Drawing for the job (mm, zero at the part's lowest x, y, z). A direction names the side the tool comes from. Give positions to 0.01 mm unless a question says otherwise; leave off trailing zeros. Write each loop counter-clockwise with the first axis right and the second up, starting at its lowest first coordinate (ties: lowest second). Pieces come first, ordered by that corner, then holes.
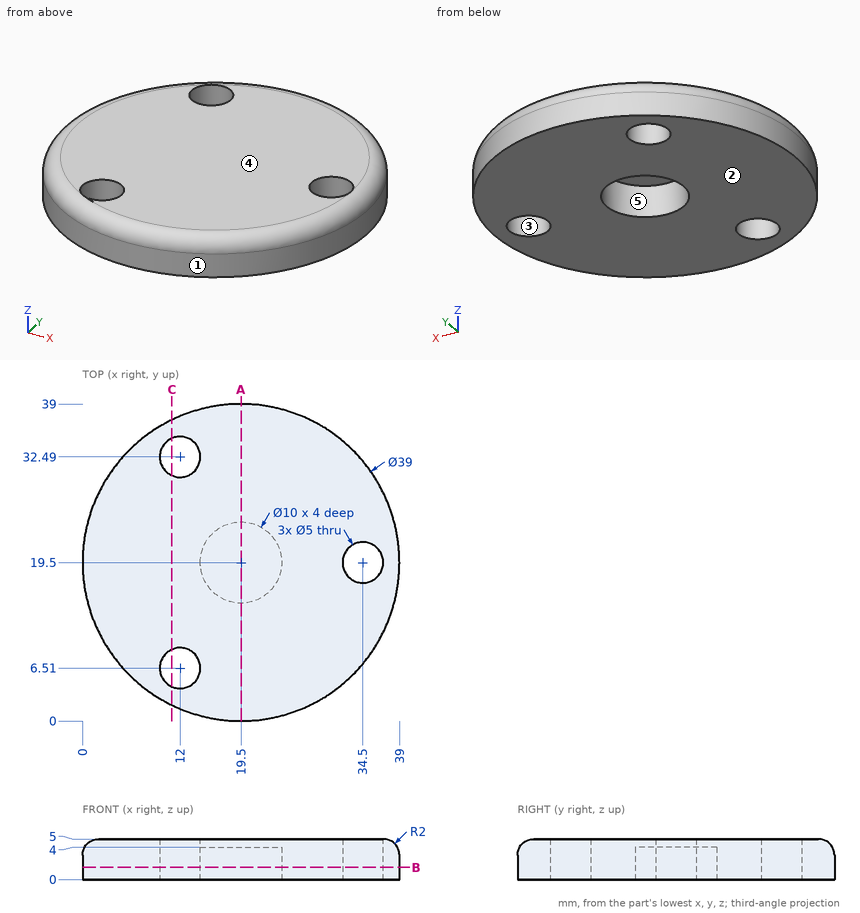
1. Pin check, flat tips, straight feed: P1, Ø4, axis at x = 12, y = 6.51, coming from the +Z side; P2, Ø3, axis at x = 12, z = 1, coming from the +Y side; P3, Ø2, axis at x = 28, z = 3.5, coming from the +Y side; P4, Ø1, axis at y = 28.5, z = 1.5, coming from the +X side. Stop position of each tip, or through.
Calculated:
P1: passes through
P2: stops at y = 38.05
P3: stops at y = 37.47
P4: stops at x = 37.05
2. Which spindle directions (+Z, -Z, +X, -X, +Y, -Y) get a long thin tool onto all of the face, cutting with end or side? Do the marked faces 4 and 5. Say none if no direction does.
Calculated:
face 4: +Z, +X, -X, +Y, -Y
face 5: -Z
3. Probe probe 1 along Y at (x, z) = (19.5, 1.3); probe 2 along X at (y, z) = (18.5, 3.6); probe 3 along Y at (x, z) = (11, 2.1). List the from-to ranges inside material, lowest first.
Calculated:
probe 1: y = 0 to 14.5, 24.5 to 39
probe 2: x = 0.12 to 14.6, 24.4 to 32.21, 36.79 to 38.88
probe 3: y = 1.95 to 4.22, 8.8 to 30.2, 34.78 to 37.05
4. Pull direction Y, two halves, no side cores. Call the marked faces 1, 2 and 3: +Y half, -Y half, draft (parallel to the pull), parting line (faces both ways), or undercut.
Calculated:
face 1: parting line
face 2: draft
face 3: undercut
5. Slice it at A-A, the plane x = 19.5. Write the cut outline in (y, z), and give its area (3 significant figures).
Calculated:
outline: (0, 0) - (14.5, 0) - (14.5, 4) - (24.5, 4) - (24.5, 0) - (39, 0) - (39, 3) arc R2 ccw to (37, 5) - (2, 5) arc R2 ccw to (0, 3) - close
area: 153 mm2
6. Slice it at C-C, the plane x = 11. State how many separate pieces and enclosed holes the cut face has, and give its area (3 significant figures).
Calculated:
separate pieces: 3
enclosed holes: 0
area: 128 mm2
7. Slice it at B-B, the plane z = 1.5. Write the cut outline in (x, y).
Calculated:
outline: circle Ø39 at (19.5, 19.5); hole circle Ø5 at (12, 6.51); hole circle Ø5 at (12, 32.49); hole circle Ø10 at (19.5, 19.5); hole circle Ø5 at (34.5, 19.5)
